Geometry: final body of the model. Coordinates: model frame, mm. Give positions to 0.01 mm unless a question says otherwise; leave off trailing zeros. Loops run counter-clockwise (first coordinate to the right, second up) from the corner with the lowest first, then second, coordinate; pieces in that order, holes last. Notation, with made-up numbers: (63, -7) - (112, -7) arc R33 ccw to (112, 25) - close; hole circle Ø4 at (0, 10). An arc over 180 degrees is marked (long way). Use CSV: the item, a comma, the result in double quotes. Start each with the question number.
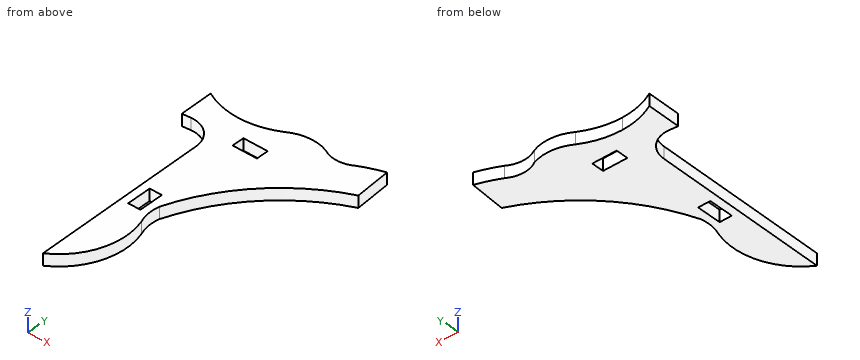
```python
from build123d import *

# Parameters (mm, degrees)
SKETCH1_W           = 1.5875
SKETCH1_H           = 3.175
SKETCH1_W_2         = 3.175
SKETCH1_H_2         = 1.5875
BOSS_EXTRUDE1_DEPTH = 1.524


with BuildPart() as part:
    # Sketch1 → Boss-Extrude1 (new body)
    with BuildSketch(Plane.XY):
        with BuildLine():
            ThreePointArc((-92.462594244, 53.392882958), (-87.259455285, 61.89953001), (-79.086960783, 67.613200697))
            Line((-79.086960783, 67.613200697), (-79.461877647, 72.269382522))
            ThreePointArc((-79.461877647, 72.269382522), (-81.010669369, 71.722343201), (-82.50335439, 71.03685123))
            ThreePointArc((-82.50335439, 71.03685123), (-84.40835406, 70.46229139), (-86.325241021, 70.995852197))
            ThreePointArc((-86.325241021, 70.995852197), (-88.879114534, 71.369944183), (-91.324996548, 70.545398299))
            ThreePointArc((-91.324996548, 70.545398299), (-93.73568856, 69.57630413), (-96.315834525, 69.270646985))
            ThreePointArc((-96.315834525, 69.270646985), (-98.648749132, 69.584935579), (-100.840653449, 70.443319727))
            Line((-100.840653449, 70.443319727), (-100.794339098, 66.125944717))
            Line((-100.794339098, 66.125944717), (-99.710350028, 66.223965922))
            ThreePointArc((-99.710350028, 66.223965922), (-97.295430394, 65.417299389), (-96.249595613, 63.095925369))
            Line((-96.249595613, 63.095925369), (-96.004020182, 40.203642412))
            ThreePointArc((-96.004020182, 40.203642412), (-92.311993967, 44.659081136), (-92.198099781, 50.444322695))
            ThreePointArc((-92.198099781, 50.444322695), (-92.555911633, 51.898369022), (-92.462594244, 53.392882958))
        make_face()
        with Locations((-94.329440184, 53.37562941)):
            Rectangle(SKETCH1_W, SKETCH1_H, mode=Mode.SUBTRACT)
        with Locations((-92.073197515, 66.344715332)):
            Rectangle(SKETCH1_W_2, SKETCH1_H_2, mode=Mode.SUBTRACT)
    extrude(amount=BOSS_EXTRUDE1_DEPTH)


solid = part.part
```
Item 1: Section A-A (z = 0.95). Give the number of separate pieces and of enclosed holes in the cut face, plus the area to 3 significant figures.
Item 2: Ray query, probe 1 along Y at (x, z) = (-92.75, 0.8); probe 2 along X at (y, z) = (52, 1.05); probe 3 along Y at (x, z) = (-94.5, 0.3). Return the intervals inside material, ascending.
Item 3: Section B-B (x = -91). Output: boundary loops of the cut face in (y, z), plus the area to 3 significant figures.
Item 4: Pin query (flat end, axial travel): pin 1 Ø0.5 at (y, z) = (52.5, 0.5) entering from +X; pin 2 Ø0.5 at (y, z) = (54, 1) entering from -X; pin 3 Ø0.8 at (x, z) = (-94.5, 0.5) entering from +Y. Return the tip coordinate at first contact, or that it passes through.
Item 5: Section D-D (x = -87). Output: boundary loops of the cut face in (y, z).
Item 6: Section C-C (y = 63.5). Output: boundary loops of the cut face in (x, z), plus the area to 3 significant figures.
Outcome:
1,separate pieces,"1"
1,enclosed holes,"2"
1,area,"227 mm2"
2,probe 1,"y = 43.67 to 65.55, 67.14 to 69.88"
2,probe 2,"x = -96.13 to -95.12, -93.54 to -92.56"
2,probe 3,"y = 41.35 to 51.79, 54.96 to 69.41"
3,outline,"(56.69, 0) - (65.55, 0) - (65.55, 1.52) - (56.69, 1.52) - close; (67.14, 0) - (70.73, 0) - (70.73, 1.52) - (67.14, 1.52) - close"
3,area,"19.0 mm2"
4,pin 1,"stops at x = -92.56"
4,pin 2,"stops at x = -96.15"
4,pin 3,"stops at y = 69.49"
5,outline,"(62.17, 0) - (71.22, 0) - (71.22, 1.52) - (62.17, 1.52) - close"
6,outline,"(-96.28, 0) - (-85.6, 0) - (-85.6, 1.52) - (-96.28, 1.52) - close"
6,area,"16.3 mm2"
